The figure shows three views and two pictorial views of one solid part (mm, origin at its lowest corner). Answer the questions. A direction names the side the tool comes from. Coordinates: 2 decimals unless noted, no trailing zeros. Order: outer loops, then holes, each group sorted by start corner. A loop starts at its lowest first (then second) coordinate and runs counter-clockwise, first axis right, second up. Notation, with made-up numbers: (52, 87.5) -> (56, 87.5) arc R19 ccw to (56, 122.5) -> close; hole circle Ø7 at (-18, 65). An arc over 180 degrees is marked (long way). Write item = value, one per line. Start each with the question number.
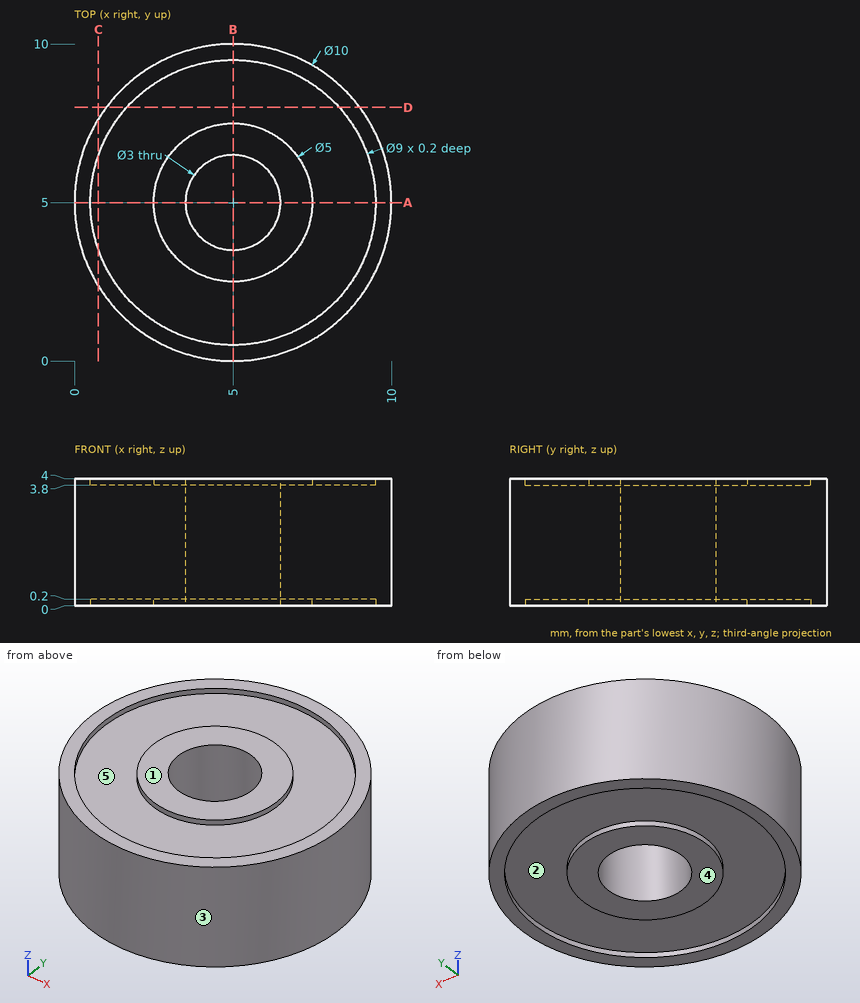
Item 1: Section A-A, the plane y = 5 is taken. Give the vertices of the cut face in (x, z), then the cut area to 3 significant figures.
Item 2: For a pull along X with two mould halves and no side action, classify the marked faces 1, 2 and 3 as pulls with the +X half, pulls with the -X half, needs draft (parallel to the pull), parting line crosses it, or undercut.
Item 3: Section C-C, the plane x = 0.75 is taken. Give the vertices of the cut face in (y, z), then the cut area to 3 significant figures.
Item 4: Consider probe 1 along Y at (x, z) = (5, 0.15); probe 2 along Y at (x, z) = (5, 2.8); probe 3 along X at (y, z) = (5.75, 0.35). Determine where each line is inside the solid, lowest interval first.
Item 5: Section D-D, the plane y = 8 is taken. Give the vertices of the cut face in (x, z).
Item 6: This flat-tipped pin is pushed along its axis until it touches: pin 1 (1 mm diameter, centred on y = 6, z = 1.5, fed in from -X). Where does it stop, or does it pass through?
Item 7: Which of the six approach directions +Z, -Z, +X, -X, +Y, -Y give full straight-line access (tool end or side, diameter ignored) to the marked faces 4 and 5?
A:
q1.outline = (0, 0) -> (0.5, 0) -> (0.5, 0.2) -> (2.5, 0.2) -> (2.5, 0) -> (3.5, 0) -> (3.5, 4) -> (2.5, 4) -> (2.5, 3.8) -> (0.5, 3.8) -> (0.5, 4) -> (0, 4) -> close; (6.5, 0) -> (7.5, 0) -> (7.5, 0.2) -> (9.5, 0.2) -> (9.5, 0) -> (10, 0) -> (10, 4) -> (9.5, 4) -> (9.5, 3.8) -> (7.5, 3.8) -> (7.5, 4) -> (6.5, 4) -> close
q1.area = 26.4 mm^2
q2.face_1 = needs draft
q2.face_2 = undercut
q2.face_3 = parting line crosses it
q3.outline = (2.37, 0) -> (3.52, 0) -> (3.52, 0.2) -> (6.48, 0.2) -> (6.48, 0) -> (7.63, 0) -> (7.63, 4) -> (6.48, 4) -> (6.48, 3.8) -> (3.52, 3.8) -> (3.52, 4) -> (2.37, 4) -> close
q3.area = 19.9 mm^2
q4.probe_1 = 0 to 0.5, 2.5 to 3.5, 6.5 to 7.5, 9.5 to 10
q4.probe_2 = 0 to 3.5, 6.5 to 10
q4.probe_3 = 0.06 to 3.7, 6.3 to 9.94
q5.outline = (1, 0) -> (1.65, 0) -> (1.65, 0.2) -> (8.35, 0.2) -> (8.35, 0) -> (9, 0) -> (9, 4) -> (8.35, 4) -> (8.35, 3.8) -> (1.65, 3.8) -> (1.65, 4) -> (1, 4) -> close
q6.pin_1 = 0.03
q7.face_4 = -Z, +X, -X, +Y, -Y
q7.face_5 = +Z
